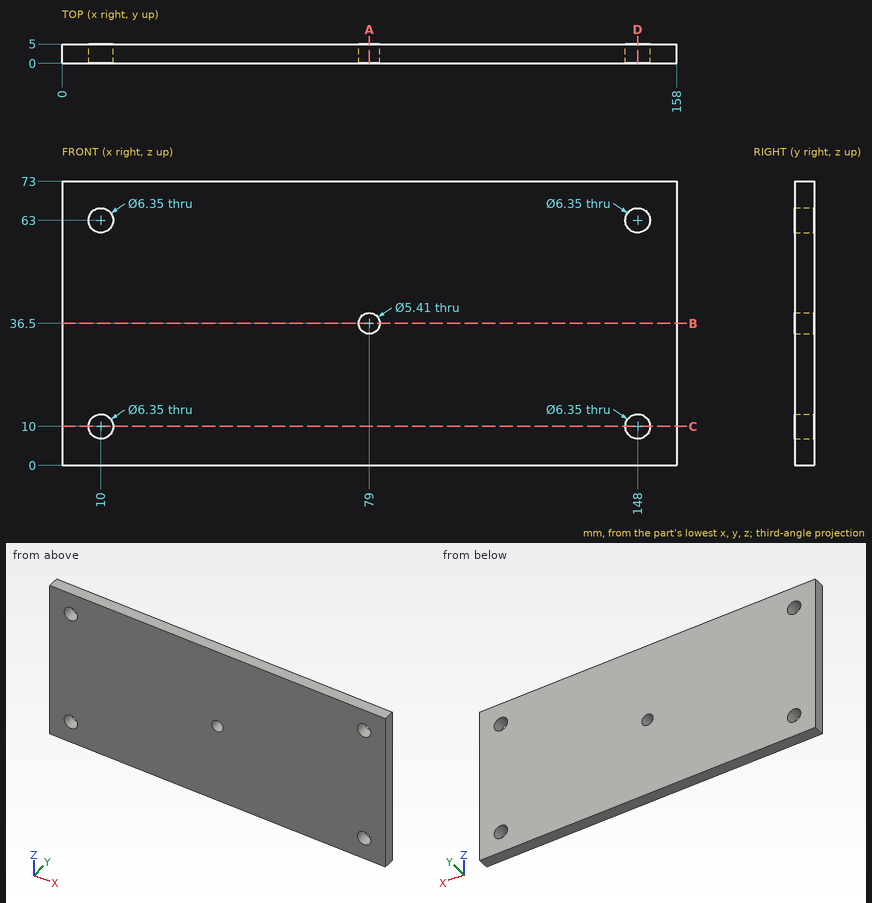
Could you check a few things on this drawing? It's one solid part, dimensions in mm from its lowest x, y, z. Round coordinates to 2 decimals unless told otherwise and drop trailing zeros. Loops run counter-clockwise (first coordinate to the right, second up) from the corner with the lowest first, then second, coordinate; pieces in that order, holes last. Notation, with made-up numbers: (46, -20) -> (99, -20) arc R31 ccw to (99, 11) -> close; hole circle Ø6 at (8, -28). An arc over 180 degrees is marked (long way). One line per item, written item: value. Start each with the question number.
1. If we section it at B-B, the plane z = 36.5: Write out the boundary of the cut face in (x, y) (1 decimal).
2. If we section it at C-C, the plane z = 10: Write out the boundary of the cut face in (x, y) (3 decimals).
3. If we section it at D-D, the plane x = 148: Write out the boundary of the cut face in (y, z) (3 decimals).
4. If I drill on probe 1 along Z at (x, y) = (148, 2.5) (3 decimals); probe 2 along X at (y, z) = (1.8, 36.5) (1 decimal); probe 3 along X at (y, z) = (3.7, 10) (3 decimals), over which ranges is the centre line in solid material (lowest first)?
5. If we section it at A-A, the plane x = 79: Write out the boundary of the cut face in (y, z) (1 decimal), then the cut area to 3 significant figures.
Calculated:
1. outline: (0, 0) -> (76.3, 0) -> (76.3, 5) -> (0, 5) -> close; (81.7, 0) -> (158, 0) -> (158, 5) -> (81.7, 5) -> close
2. outline: (0, 0) -> (6.825, 0) -> (6.825, 5) -> (0, 5) -> close; (13.175, 0) -> (144.825, 0) -> (144.825, 5) -> (13.175, 5) -> close; (151.175, 0) -> (158, 0) -> (158, 5) -> (151.175, 5) -> close
3. outline: (0, 0) -> (5, 0) -> (5, 6.825) -> (0, 6.825) -> close; (0, 13.175) -> (5, 13.175) -> (5, 59.825) -> (0, 59.825) -> close; (0, 66.175) -> (5, 66.175) -> (5, 73) -> (0, 73) -> close
4. probe 1: z = 0 to 6.825, 13.175 to 59.825, 66.175 to 73
4. probe 2: x = 0 to 76.3, 81.7 to 158
4. probe 3: x = 0 to 6.825, 13.175 to 144.825, 151.175 to 158
5. outline: (0, 0) -> (5, 0) -> (5, 33.8) -> (0, 33.8) -> close; (0, 39.2) -> (5, 39.2) -> (5, 73) -> (0, 73) -> close
5. area: 338 mm²
